from build123d import *

# Parameters (mm, degrees)
BOSS_EXTRUDE1_DEPTH                             = 45
SKETCH3_R                                       = 13.7
CUT_EXTRUDE1_DEPTH                              = 3
CSK_FOR_M3_FLAT_HEAD_MACHINE_SCREW4_AT_2_COUNT  = 2
CSK_FOR_M3_FLAT_HEAD_MACHINE_SCREW4_AT_2_PITCH  = 24
CSK_FOR_M3_FLAT_HEAD_MACHINE_SCREW4_AT_3_COUNT  = 2
CSK_FOR_M3_FLAT_HEAD_MACHINE_SCREW4_AT_3_PITCH  = 33.941125497
CSK_FOR_M3_FLAT_HEAD_MACHINE_SCREW4_AT_4_COUNT  = 2
CSK_FOR_M3_FLAT_HEAD_MACHINE_SCREW4_AT_4_PITCH  = 24
SKETCH10_R                                      = 7.25
CUT_EXTRUDE2_DEPTH                              = 69.23672032
SKETCH15_R                                      = 48.495489481
SKETCH15_R_2                                    = 44
CUT_EXTRUDE4_DEPTH                              = 70.822990483
SKETCH11_R                                      = 10.5
CUT_EXTRUDE3_DEPTH                              = 2
CBORE_FOR_M5_HEX_HEAD_BOLT1_D                   = 3.4
CBORE_FOR_M5_HEX_HEAD_BOLT1_CBORE_D             = 5.3
CBORE_FOR_M5_HEX_HEAD_BOLT1_CBORE_DEPTH         = 4
BOSS_EXTRUDE6_DEPTH                             = 1.5875
BOSS_EXTRUDE6_DEPTH_BACK                        = 1.5875
SKETCH28_W                                      = 50.8
SKETCH28_H                                      = 100
FILLET4_R                                       = 9
CSK_FOR_M3_FLAT_HEAD_MACHINE_SCREW3_D           = 3.4
CSK_FOR_M3_FLAT_HEAD_MACHINE_SCREW3_CSINK_D     = 6.3
CSK_FOR_M3_FLAT_HEAD_MACHINE_SCREW3_CSINK_ANGLE = 90
SKETCH32_W                                      = 50.8
SKETCH32_H                                      = 4.780360426
CUT_EXTRUDE5_DEPTH                              = 3.175


with BuildPart() as part:
    # Sketch1 → Boss-Extrude1 (new body)
    with BuildSketch(Plane.XY):
        Polygon((-37.5, 0), (-27.038942926, 0), (-15, 32), (15, 32), (27.038942926, 0), (37.5, 0), (37.5, 5), (30.5, 5), (18.084840108, 38), (-18.084840108, 38), (-30.5, 5), (-37.5, 5), align=None)
    extrude(amount=BOSS_EXTRUDE1_DEPTH)

    # Sketch3 → Cut-Extrude1 (cut)
    with BuildSketch(Plane(origin=(0, 38, 0), x_dir=(1, 0, 0), z_dir=(0, 1, 0))):
        with Locations(Location((0, -30, 0), (0, 0, 180))):
            Circle(SKETCH3_R)
    extrude(amount=-CUT_EXTRUDE1_DEPTH, mode=Mode.SUBTRACT)

    # Sketch6 → CSK for M3 Flat Head Machine Screw4 (revolve, cut)
    with BuildSketch(Plane(origin=(-12, 32, 42), x_dir=(0, 0, -1), z_dir=(1, 0, 0))):
        Polygon((0, 0), (0, 6), (1.7, 6), (1.7, 1.45), (3.15, 0), align=None)
    csk_for_m3_flat_head_machine_screw4 = revolve(axis=Axis((-12, 25.65, 42), (0, 1, 0)), mode=Mode.SUBTRACT)

    # CSK for M3 Flat Head Machine Screw4 at 2: CSK for M3 Flat Head Machine Screw4 ×2
    with Locations(*[(i * CSK_FOR_M3_FLAT_HEAD_MACHINE_SCREW4_AT_2_PITCH, 0, 0) for i in range(1, CSK_FOR_M3_FLAT_HEAD_MACHINE_SCREW4_AT_2_COUNT)]):
        add(csk_for_m3_flat_head_machine_screw4, mode=Mode.SUBTRACT)

    # CSK for M3 Flat Head Machine Screw4 at 3: CSK for M3 Flat Head Machine Screw4 ×2
    with Locations(*[Vector(0.7071067811865476, 0, -0.7071067811865475) * (i * CSK_FOR_M3_FLAT_HEAD_MACHINE_SCREW4_AT_3_PITCH) for i in range(1, CSK_FOR_M3_FLAT_HEAD_MACHINE_SCREW4_AT_3_COUNT)]):
        add(csk_for_m3_flat_head_machine_screw4, mode=Mode.SUBTRACT)

    # CSK for M3 Flat Head Machine Screw4 at 4: CSK for M3 Flat Head Machine Screw4 ×2
    with Locations(*[(0, 0, -i * CSK_FOR_M3_FLAT_HEAD_MACHINE_SCREW4_AT_4_PITCH) for i in range(1, CSK_FOR_M3_FLAT_HEAD_MACHINE_SCREW4_AT_4_COUNT)]):
        add(csk_for_m3_flat_head_machine_screw4, mode=Mode.SUBTRACT)

    # Sketch10 → Cut-Extrude2 (cut, through all)
    with BuildSketch(Plane(origin=(0, 35, 0), x_dir=(1, 0, 0), z_dir=(0, 1, 0))):
        with Locations(Location((0, -30, 0), (0, 0, 180))):
            Circle(SKETCH10_R)
    extrude(amount=-CUT_EXTRUDE2_DEPTH, mode=Mode.SUBTRACT)

    # Sketch15 → Cut-Extrude4 (cut, through all)
    with BuildSketch(Plane(origin=(0, 38, 0), x_dir=(1, 0, 0), z_dir=(0, 1, 0))):
        with Locations((0, -14.25)):
            Circle(SKETCH15_R)
        with Locations((0, -14.25)):
            Circle(SKETCH15_R_2, mode=Mode.SUBTRACT)
    extrude(amount=-CUT_EXTRUDE4_DEPTH, mode=Mode.SUBTRACT)

    # Sketch11 → Cut-Extrude3 (cut)
    with BuildSketch(Plane.XZ.offset(-32)):
        with Locations((0, 30)):
            Circle(SKETCH11_R)
    extrude(amount=-CUT_EXTRUDE3_DEPTH, mode=Mode.SUBTRACT)

    # CBORE for M5 Hex Head Bolt1 (through all)
    with Locations(Plane(origin=(0, 5, 0), x_dir=(-1, 0, 0), z_dir=(0, 1, 0))):
        with Locations((34, 35.5), (34, 3.5), (-34, 3.5), (-34, 35.5)):
            CounterBoreHole(CBORE_FOR_M5_HEX_HEAD_BOLT1_D / 2, CBORE_FOR_M5_HEX_HEAD_BOLT1_CBORE_D / 2, CBORE_FOR_M5_HEX_HEAD_BOLT1_CBORE_DEPTH)

    # Sketch28 → Boss-Extrude6 (add, two sides: drawn at the far end of the back side and taken through both)
    with BuildSketch(Plane(origin=(-18.084840108, 0, 0), x_dir=(0, 0, -1), z_dir=(1, 0, 0)).offset(-BOSS_EXTRUDE6_DEPTH_BACK)):
        with Locations((-14.25, 79)):
            Rectangle(SKETCH28_W, SKETCH28_H)
    extrude(amount=BOSS_EXTRUDE6_DEPTH + BOSS_EXTRUDE6_DEPTH_BACK)

    # Fillet4
    # the kernel refuses this fillet: 9 mm, written as the material it adds along each edge
    with BuildSketch(Plane(origin=(-16.497340108, 29, 0), x_dir=(0, -1, 0), z_dir=(-1, 0, 0))) as fillet4_piece_1_section:
        with BuildLine():
            CenterArc((FILLET4_R, -FILLET4_R), FILLET4_R, 90, 90)
            Line((0, -FILLET4_R), (0, 0))
            Line((0, 0), (FILLET4_R, 0))
        make_face()
    fillet4_piece_1 = extrude(amount=3.175, mode=Mode.PRIVATE)
    fillet4_piece_1 = split(fillet4_piece_1, bisect_by=Plane(origin=(-16.91095331, 26.920608371, -2.290762679), z_dir=(-0.9359541711547182, 0.35212183899622657, 0)), keep=Keep.TOP, mode=Mode.PRIVATE)
    add(fillet4_piece_1)

    # CSK for M3 Flat Head Machine Screw3 (through all)
    with Locations(Plane(origin=(-16.497340108, 0, 0), x_dir=(0, 0, -1), z_dir=(1, 0, 0))):
        with Locations((6.05, 49.9), (-34.55, 49.9), (-34.55, 113.1), (6.05, 113.1)):
            CounterSinkHole(CSK_FOR_M3_FLAT_HEAD_MACHINE_SCREW3_D / 2, CSK_FOR_M3_FLAT_HEAD_MACHINE_SCREW3_CSINK_D / 2, counter_sink_angle=CSK_FOR_M3_FLAT_HEAD_MACHINE_SCREW3_CSINK_ANGLE)

    # Sketch32 → Cut-Extrude5 (cut)
    with BuildSketch(Plane.ZY.offset(19.672340108)):
        with Locations((14.25, 31.390180213)):
            Rectangle(SKETCH32_W, SKETCH32_H)
    extrude(amount=CUT_EXTRUDE5_DEPTH, mode=Mode.SUBTRACT)


solid = part.part
Verification items for the finished model (mm, model axes). A direction names the side the tool comes from. Give positions to 0.01 mm unless a question says otherwise; leave off trailing zeros. Loops run counter-clockwise (first coordinate to the right, second up) from the corner with the lowest first, then second, coordinate; pieces in that order, holes last.
1) Sectioned sample at B-B, the plane x = 0. Enter the section's corners in (y, z), then the cut area to 3 significant figures.
2) Sectioned sample at D-D, the plane x = 34. Enter the section's corners in (y, z), then the cut area to 3 significant figures.
3) Depth check by flat-ended pin: pin 1 Ø4.5 at (x, z) = (12, 18) entering from +Y; pin 2 Ø12 at (x, z) = (-2.5, 32.5) entering from +Y; pin 3 Ø3.5 at (x, z) = (35.5, 29.5) entering from +Y. Enter the tip coordinate at first touch or a pass-through.
4) Thickness scan on line 1 along Z through (x, y) = (-34, 2); line 2 along Z through (x, y) = (34, 0.75); line 3 along X through (y, z) = (2, 35). Record the ranges inside material, lowest first.
5) Draft check along X on faces 3 (the flat face through (24.38, 21.27, 22.18)), 4 (the cylindrical face through (-32.047, 3.028, 37.291)), 5 (the flat face through (-25.585, 18.064, 22.185)). Enter one of: pulls with the +X half, pulls with the -X half, needs draft (parallel to the pull), parting line crosses it, or undercut.
6) Sectioned sample at A-A, the plane z = 3.5. Count the separate pieces of the cut face and the enclosed holes in it, then the cut area to 3 significant figures.
7) Sectioned sample at C-C, the plane y = 16.5. Enter the section's corners in (x, z), then the cut area to 3 significant figures.
8) Set-up check for faces 1 (the flat face through (-36, 1, 36)), 2 (the cylindrical face through (11.93, 35.69, 19.7)): record each of +Z, -Z, +X, -X, +Y, -Y from which the full face is reachable in a straight line by a thin tool's end or side.
Answers:
1. outline: (32, 0) - (38, 0) - (38, 16.3) - (35, 16.3) - (35, 22.75) - (34, 22.75) - (34, 19.5) - (32, 19.5) - close; (32, 40.5) - (34, 40.5) - (34, 37.25) - (35, 37.25) - (35, 43.7) - (38, 43.7) - (38, 45) - (32, 45) - close
1. area: 131 mm2
2. outline: (0, 0) - (5, 0) - (5, 0.85) - (1, 0.85) - (1, 1.8) - (0, 1.8) - close; (0, 5.2) - (1, 5.2) - (1, 6.15) - (5, 6.15) - (5, 32.85) - (1, 32.85) - (1, 33.8) - (0, 33.8) - close; (0, 37.2) - (1, 37.2) - (1, 38.15) - (5, 38.15) - (5, 42.18) - (0, 42.18) - close
2. area: 162 mm2
3. pin 1: stops at y = 38
3. pin 2: stops at y = 35
3. pin 3: stops at y = 5
4. line 1: z = 0 to 0.85, 6.15 to 32.85, 38.15 to 42.18
4. line 2: z = 0 to 1.8, 5.2 to 33.8, 37.2 to 42.18
4. line 3: x = -37.5 to -36.6, -31.4 to -26.29, 26.29 to 31.4, 36.6 to 37.5
5. face 3: pulls with the +X half
5. face 4: undercut
5. face 5: pulls with the -X half
6. separate pieces: 3
6. enclosed holes: 0
6. area: 872 mm2
7. outline: (-26.17, 0) - (-20.83, 0) - (-20.83, 45) - (-26.17, 45) - close; (20.83, 0) - (26.17, 0) - (26.17, 45) - (20.83, 45) - close
7. area: 481 mm2
8. face 1: +Y
8. face 2: +Y, -Y
